```python
from build123d import *

# Parameters (mm, degrees)
SKETCH133_W     = 15
SKETCH133_H     = 10
PAD068_DEPTH    = 7
SKETCH134_W     = 9.2
SKETCH134_H     = 6.2
POCKET056_DEPTH = 14
SKETCH135_W     = 2
SKETCH135_H     = 2
POCKET057_DEPTH = 5


with BuildPart() as part:
    # Sketch133 → Pad068 (new body)
    with BuildSketch(Plane.XY):
        Rectangle(SKETCH133_W, SKETCH133_H)
    extrude(amount=PAD068_DEPTH)

    # Sketch134 (on Face4 of Pad068) → Pocket056 (cut)
    with BuildSketch(Plane(origin=(-7.5, 0, 0), x_dir=(0, -1, 0), z_dir=(-1, 0, 0))):
        with Locations((0, 3.5)):
            Rectangle(SKETCH134_W, SKETCH134_H)
    extrude(amount=-POCKET056_DEPTH, mode=Mode.SUBTRACT)

    # Sketch135 (on Face3 of Pocket056) → Pocket057 (cut)
    with BuildSketch(Plane.YZ.offset(7.5)):
        with Locations((0, 3.5)):
            Rectangle(SKETCH135_W, SKETCH135_H)
    extrude(amount=-POCKET057_DEPTH, mode=Mode.SUBTRACT)


with BuildPart() as part_1:
    # Body009 placement: moved
    add(part.part.moved(Location((-20, 11, 2))))


solid = part_1.part
```
The listing builds one solid part. Answer for the finished solid, in the listing's coordinates (mm). A direction names the side the tool comes from. Coordinates: 2 decimals unless noted, no trailing zeros. Loops run counter-clockwise (first coordinate to the right, second up) from the corner with the lowest first, then second, coordinate; pieces in that order, holes last. Notation, with made-up numbers: (14, 6) -> (31, 6) arc R21 cw to (31, 39) -> close; hole circle Ø3 at (68, 22.5). An arc over 180 degrees is marked (long way). Use one line per item in the form item = value. Start each with the question number.
Item 1: Consider L1, parallel to Y at x = -17.25, z = 4; L2, parallel to Z at x = -20.25, y = 14.25; L3, parallel to X at y = 11, z = 3.5. Determine where each line is inside the solid, lowest interval first. Write a range as [from, to].
Item 2: The part is cut by section C-C on x = -16.25. Determine the outline of the cut face in (y, z), then the cut area to 3 significant figures.
Item 3: The mould has two halves that part along Y. Classify faces 1 (the face through (-21, 11, 8.6)), 2 (the face through (-20, 16, 5)), 3 (the face through (-21, 6.4, 5)), 4 (the face through (-20, 11, 2)): released by +Y, released by -Y, zero draft, split by the parting line, or undercut.
Item 4: The part is cut by section A-A on y = 11.5. Determine the outline of the cut face in (x, z), then the cut area to 3 significant figures.
Item 5: The part is cut by section B-B on z = 5.75. Determine the outline of the cut face in (x, y), then the cut area to 3 significant figures.
Item 6: A flat-ended cylindrical pin translates along its axis: pin 1 Ø1.5 at (y, z) = (11, 5) entering from -X. Find the tip coordinate at first contact, or state that the pin passes through.
Item 7: A tool of negligible diameter and unlimited length cuts with its end or side. For faces 5 (the face through (-21, 15.6, 5)), 6 (the face through (-13, 11, 4.5)), 7 (the face through (-20, 6, 5)), from which of +Z, -Z, +X, -X, +Y, -Y can it reach the whole face along a straight path? Write none if from no direction.
Item 8: The part is cut by section D-D on y = 8. Determine the outline of the cut face in (x, z).
Answer key:
q1.L1 = [6, 6.4], [15.6, 16]
q1.L2 = [2, 2.4], [8.6, 9]
q1.L3 = [-13.5, -12.5]
q2.outline = (6, 2) -> (16, 2) -> (16, 9) -> (6, 9) -> close; hole (6.4, 2.4) -> (15.6, 2.4) -> (15.6, 8.6) -> (6.4, 8.6) -> close
q2.area = 13.0 mm2
q3.face_1 = undercut
q3.face_2 = released by +Y
q3.face_3 = undercut
q3.face_4 = zero draft
q4.outline = (-27.5, 2) -> (-12.5, 2) -> (-12.5, 4.5) -> (-13.5, 4.5) -> (-13.5, 2.4) -> (-27.5, 2.4) -> close; (-27.5, 8.6) -> (-13.5, 8.6) -> (-13.5, 6.5) -> (-12.5, 6.5) -> (-12.5, 9) -> (-27.5, 9) -> close
q4.area = 16.2 mm2
q5.outline = (-27.5, 6) -> (-12.5, 6) -> (-12.5, 10) -> (-13.5, 10) -> (-13.5, 6.4) -> (-27.5, 6.4) -> close; (-27.5, 15.6) -> (-13.5, 15.6) -> (-13.5, 12) -> (-12.5, 12) -> (-12.5, 16) -> (-27.5, 16) -> close
q5.area = 19.2 mm2
q6.pin_1 = -13.5
q7.face_5 = -X
q7.face_6 = +X, -X
q7.face_7 = +Z, -Z, +X, -X, -Y
q8.outline = (-27.5, 2) -> (-12.5, 2) -> (-12.5, 9) -> (-27.5, 9) -> (-27.5, 8.6) -> (-13.5, 8.6) -> (-13.5, 2.4) -> (-27.5, 2.4) -> close
